Drawing for the job (mm, zero at the part's lowest x, y, z). A direction names the side the tool comes from. Give positions to 0.01 mm unless a question says otherwise; leave off trailing zeros. Write each loop counter-clockwise with the first axis right and the second up, starting at its lowest first coordinate (ties: lowest second). Pieces come first, ordered by that corner, then holes.
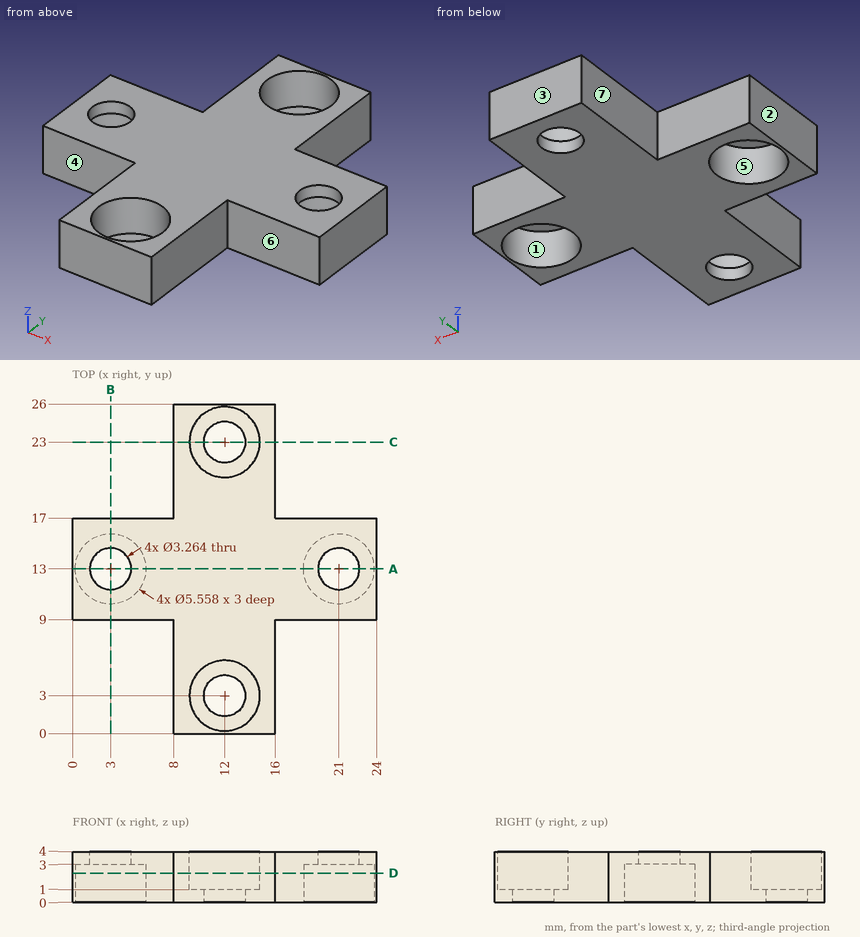
1. Pull direction Y, two halves, no side cores. Call the marked faces 1, 2 and 3: +Y half, -Y half, draft (parallel to the pull), parting line (faces both ways), or undercut.
Calculated:
face 1: undercut
face 2: draft
face 3: +Y half
2. Slice it at A-A, the plane y = 13. Write the cut outline in (x, z).
Calculated:
outline: (0, 0) - (0.22, 0) - (0.22, 3) - (1.37, 3) - (1.37, 4) - (0, 4) - close; (4.63, 3) - (5.78, 3) - (5.78, 0) - (18.22, 0) - (18.22, 3) - (19.37, 3) - (19.37, 4) - (4.63, 4) - close; (22.63, 3) - (23.78, 3) - (23.78, 0) - (24, 0) - (24, 4) - (22.63, 4) - close
3. Which spindle directions (+Z, -Z, +X, -X, +Y, -Y) get a long thin tool onto all of the face, cutting with end or side? Do the marked faces 4, 5, 6 and 7. Say none if no direction does.
Calculated:
face 4: +Z, -Z, -X, -Y
face 5: -Z
face 6: +Z, -Z, +X, -Y
face 7: +Z, -Z, -X, +Y
4. Slice it at B-B, the plane x = 3. Write the cut outline in (y, z).
Calculated:
outline: (9, 0) - (10.22, 0) - (10.22, 3) - (11.37, 3) - (11.37, 4) - (9, 4) - close; (14.63, 3) - (15.78, 3) - (15.78, 0) - (17, 0) - (17, 4) - (14.63, 4) - close
5. Slice it at C-C, the plane y = 23. Write the cut outline in (x, z).
Calculated:
outline: (8, 0) - (10.37, 0) - (10.37, 1) - (9.22, 1) - (9.22, 4) - (8, 4) - close; (13.63, 0) - (16, 0) - (16, 4) - (14.78, 4) - (14.78, 1) - (13.63, 1) - close
6. Probe probe 1 along Y at (x, z) = (12, 2.4); probe 2 along Y at (x, z) = (14.25, 2.9); probe 3 along Y at (x, z) = (21, 3.75). List the from-to ranges inside material, lowest first.
Calculated:
probe 1: y = 0 to 0.22, 5.78 to 20.22, 25.78 to 26
probe 2: y = 0 to 1.37, 4.63 to 21.37, 24.63 to 26
probe 3: y = 9 to 11.37, 14.63 to 17
7. Slice it at D-D, the plane z = 2.3. Write the cut outline in (x, y).
Calculated:
outline: (0, 9) - (8, 9) - (8, 0) - (16, 0) - (16, 9) - (24, 9) - (24, 17) - (16, 17) - (16, 26) - (8, 26) - (8, 17) - (0, 17) - close; hole circle Ø5.56 at (3, 13); hole circle Ø5.56 at (12, 3); hole circle Ø5.56 at (12, 23); hole circle Ø5.56 at (21, 13)
8. Pin check, flat tips, straight feed: P1, Ø2, axis at y = 21, z = 2, coming from the -X side; P2, Ø1.2, axis at y = 3, z = 3, coming from the +X side; P3, Ø4.5, axis at x = 3, y = 13, coming from the -Z side; P4, Ø1, axis at x = 11.5, y = 23, coming from the +Z side. Stop position of each tip, or through.
Calculated:
P1: stops at x = 8
P2: stops at x = 16
P3: stops at z = 3
P4: passes through
